from build123d import *

# Parameters (mm, degrees)
F0_W     = 38.1
F0_H     = 76.2
F1_DEPTH = 2.54
F2_D     = 3.2512
F2_DEPTH = 14.605
F2_TIP   = 0.9767590223
F3_R     = 2.54


with BuildPart() as f1:
    # F0 (on Top) → F1 (new body)
    with BuildSketch(Plane.XY):
        Rectangle(F0_W, F0_H)
    extrude(amount=F1_DEPTH)

    # F2
    with Locations(Plane(origin=(0, 0, 0), x_dir=(1, 0, 0), z_dir=(0, 0, -1))):
        with Locations((-14.605, -33.655), (14.605, -33.655), (14.605, 33.655), (-14.605, 33.655)):
            Hole(F2_D / 2, depth=F2_DEPTH)
            with Locations((0, 0, -(F2_DEPTH + F2_TIP / 2))):  # 118° drill point
                Cone(0, F2_D / 2, F2_TIP, mode=Mode.SUBTRACT)

    # F3
    f3_edges = [f1.edges().sort_by_distance(p)[0] for p in [
        (-19.05, 38.1, 1.27),
        (-19.05, -38.1, 1.27),
        (19.05, 38.1, 1.27),
        (19.05, -38.1, 1.27),
    ]]
    fillet(f3_edges, radius=F3_R)


solid = f1.part
Geometry check sheet. Reference: the model listing, model coordinates, mm. Give positions to 0.01 mm unless a question says otherwise; leave off trailing zeros. Loops run counter-clockwise (first coordinate to the right, second up) from the corner with the lowest first, then second, coordinate; pieces in that order, holes last.
(1) Section check A-A on x = -14.5. Record the cut outline in (y, z), then the cut area to 3 significant figures.
From the geometry:
outline: (-38.1, 0) - (-35.28, 0) - (-35.28, 2.54) - (-38.1, 2.54) - close; (-32.03, 0) - (32.03, 0) - (32.03, 2.54) - (-32.03, 2.54) - close; (35.28, 0) - (38.1, 0) - (38.1, 2.54) - (35.28, 2.54) - close
area: 177 mm2
(2) Thickness scan on L1, parallel to Y at x = 17, z = 1.95. Record the ranges inside material, lowest first.
From the geometry:
L1: y = -38.05 to 38.05
(3) Release check for a two-part mould opening along X. For faces 1 (the cylindrical face through (-14.25, 35.24, 1.29)), 2 (the flat face through (19.05, 0, 1)), 3 (the cylindrical face through (-18.326, 37.336, 1.288)) record: released by +X, released by -X, zero draft, split by the parting line, or undercut.
From the geometry:
face 1: undercut
face 2: released by +X
face 3: released by -X
